from build123d import *

# Parameters (mm, degrees)
F1_DEPTH      = 25.4
F1_DEPTH_BACK = 25.4
F2_DEPTH      = 5.08
F2_DEPTH_BACK = 5.08
F0_R          = 12.5
F3_DEPTH      = 25.4
F3_DEPTH_BACK = 25.4


# Not quite as in the source:
# - ends of sketch curves that miss each other by under 0.0002 mm in the source are joined


with BuildPart() as f1:
    # F0 (on Top) → F1 (new body, two sides)
    with BuildSketch(Plane.XY) as f1_sk:
        with BuildLine():
            ThreePointArc((-141.983922, -7.818031), (-146.8508026584, 3.2418013861), (-158.2932409879, 7.1247158622))
            ThreePointArc((-158.2932409879, 7.1247158622), (-168.0437543861, 2.3150883416), (-171.983922, -7.818031))
            ThreePointArc((-171.983922, -7.818031), (-168.0616462811, -17.9315874838), (-158.3460520332, -22.7560563639))
            ThreePointArc((-158.3460520332, -22.7560563639), (-146.8703655162, -18.8957552811), (-141.983922, -7.818031))
        make_face()
        with BuildLine():
            ThreePointArc((-146.983922, -7.818031), (-156.983922, -17.818031), (-166.983922, -7.818031))
            ThreePointArc((-166.983922, -7.818031), (-156.983922, 2.181969), (-146.983922, -7.818031))
        make_face(mode=Mode.SUBTRACT)
    extrude(amount=F1_DEPTH)
    extrude(f1_sk.sketch, amount=-F1_DEPTH_BACK)

    # F0 (on Top) → F2 (join, two sides)
    with BuildSketch(Plane.XY) as f2_sk:
        with BuildLine():
            ThreePointArc((-102.6737479638, -27.8325586075), (-120.8349111956, -7.8810440571), (-102.601594983, 12.004552808))
            Line((-102.601594983, 12.004552808), (-158.293241, 7.124716))
            ThreePointArc((-158.293241, 7.124716), (-146.8508026584, 3.2418013861), (-141.983922, -7.818031))
            ThreePointArc((-141.983922, -7.818031), (-146.8703655162, -18.8957552811), (-158.3460520332, -22.7560563639))
            Line((-158.3460520332, -22.7560563639), (-102.6737479638, -27.8325586075))
        make_face()
    extrude(amount=F2_DEPTH)
    extrude(f2_sk.sketch, amount=-F2_DEPTH_BACK)

    # F0 (on Top) → F3 (join, two sides)
    with BuildSketch(Plane.XY) as f3_sk:
        with BuildLine():
            ThreePointArc((-102.6737479638, -27.8325586075), (-87.3585958165, -22.6952258981), (-80.834944, -7.917268))
            ThreePointArc((-80.834944, -7.917268), (-87.3318521255, 6.8362573357), (-102.601594983, 12.004552808))
            ThreePointArc((-102.601594983, 12.004552808), (-120.8349111956, -7.8810440571), (-102.6737479638, -27.8325586075))
        make_face()
        with Locations((-100.834944, -7.917268)):
            Circle(F0_R, mode=Mode.SUBTRACT)
    extrude(amount=F3_DEPTH)
    extrude(f3_sk.sketch, amount=-F3_DEPTH_BACK)


solid = f1.part
Part model, mm, in its own coordinate system. Coordinates: 2 decimals unless noted, no trailing zeros. Write each loop counter-clockwise with the first axis right and the second up, starting at its lowest first coordinate (ties: lowest second). Pieces come first, ordered by that corner, then holes. Notation, with made-up numbers: M 3,37 L 52,37 A14 ccw 52,63 Z; hole C -26.5,73 d11. An arc over 180 degrees is marked long. Return JSON: item names as keys, results as strings.
1. Flat gauge pins, fed straight in: pin 1 Ø18 at (x, y) = (-156.98, -7.82) entering from -Z; pin 2 Ø1.5 at (x, y) = (-126.5, 2.5) entering from +Z; pin 3 Ø6 at (y, z) = (1.5, 14) entering from -X; pin 4 Ø10 at (y, z) = (-18, 0) entering from -X. Where does each tip first touch, or does it go through?
Determined:
{"pin 1": "through", "pin 2": "z = 5.08", "pin 3": "x = -170.59", "pin 4": "x = -171.06"}
2. Probe L1, parallel to X at y = -8, z = -20.5; L2, parallel to X at y = -3, z = -22.5; L3, parallel to X at y = -18.5, z = 14. List the from-to ranges inside material, lowest first.
Determined:
{"L1": "-171.98 to -166.98, -146.99 to -141.99, -120.83 to -113.33, -88.34 to -80.84", "L2": "-171.19 to -165.75, -148.22 to -142.78, -120.22 to -112.33, -89.34 to -81.45", "L3": "-167.51 to -146.45, -117.81 to -107.49, -94.18 to -83.86"}
3. Saw through at C-C, the plane x = -154.5. Write the cut outline in (y, z).
Determined:
{"outline": "M -23.11,-5.08 L -22.61,-5.08 L -22.61,-25.4 L -17.5,-25.4 L -17.5,25.4 L -22.61,25.4 L -22.61,5.08 L -23.11,5.08 Z; M 1.87,-25.4 L 6.97,-25.4 L 6.97,-5.08 L 7.46,-5.08 L 7.46,5.08 L 6.97,5.08 L 6.97,25.4 L 1.87,25.4 Z"}
4. Saw through at D-D, the plane y = -5.5. Write the cut outline in (x, z), then the cut area to 3 significant figures.
Determined:
{"outline": "M -171.8,-25.4 L -166.71,-25.4 L -166.71,25.4 L -171.8,25.4 Z; M -147.26,-25.4 L -142.16,-25.4 L -142.16,-5.08 L -120.69,-5.08 L -120.69,-25.4 L -113.1,-25.4 L -113.1,25.4 L -120.69,25.4 L -120.69,5.08 L -142.16,5.08 L -142.16,25.4 L -147.26,25.4 Z; M -88.57,-25.4 L -80.98,-25.4 L -80.98,25.4 L -88.57,25.4 Z", "area": "1,510 mm²"}
5. Saw through at A-A, the plane z = -8. Write the cut outline in (x, y), then the cut area to 3 significant figures.
Determined:
{"outline": "C -156.98,-7.82 d30; C -100.83,-7.92 d40; hole C -156.98,-7.82 d20; hole C -100.83,-7.92 d25", "area": "1,160 mm²"}
6. Pull direction X, two halves, no side cores. Call faces 1 (the face through (-131, -8, -5.08)), 2 (the face through (-130.9, -25.26, 0.07)), 3 (the face through (-131, -8, 5.08)), 4 (the face through (-110, -17, -25.4)): pulls with the +X half, pulls with the -X half, needs draft (parallel to the pull), parting line crosses it, or undercut.
Determined:
{"face 1": "undercut", "face 2": "pulls with the -X half", "face 3": "undercut", "face 4": "needs draft"}
7. Saw through at B-B, the plane z = 2.5. Write the cut outline in (x, y).
Determined:
{"outline": "M -158.35,-22.76 L -102.67,-27.83 A20 ccw long -102.6,12 L -158.29,7.12 A15 ccw Z; hole C -156.98,-7.82 d20; hole C -100.83,-7.92 d25"}
